Geometry: final body of the model. Coordinates: model frame, mm. A direction names the side the tool comes from. Coordinates: 2 decimals unless noted, no trailing zeros. Loops run counter-clockwise (first coordinate to the right, second up) from the corner with the lowest first, then second, coordinate; pieces in that order, holes last. Notation, with made-up numbers: (64, 73.5) -> (116, 73.5) arc R18 cw to (116, 77.5) -> close; hole circle Ø11 at (13, 89). An arc over 180 degrees is marked (long way). One line per item, written item: value. Start each with the question number.
from build123d import *

# Parameters (mm, degrees)
BOSS_EXTRUDE1_DEPTH                                  = 38.1
CBORE_FOR_3_8_BINDING_HEAD_MACHINE_SCREW_D           = 10.0838
CBORE_FOR_3_8_BINDING_HEAD_MACHINE_SCREW_CBORE_D     = 20.6375
CBORE_FOR_3_8_BINDING_HEAD_MACHINE_SCREW_CBORE_DEPTH = 3.175
FILLET1_R                                            = 2.54
FILLET2_R                                            = 6.35


with BuildPart() as part:
    # Sketch1 → Boss-Extrude1 (new body)
    with BuildSketch(Plane.XY):
        Polygon((0, 0), (44.45, 0), (44.45, -9.525), (-38.1608076, -9.525), (-38.1608076, 0), (-12.7608076, 0), (-6.35, 44.45), (0, 44.45), align=None)
    extrude(amount=BOSS_EXTRUDE1_DEPTH)

    # CBORE for 3/8 Binding Head Machine Screw1 (through all)
    with Locations(Plane(origin=(0, 0, 0), x_dir=(1, 0, 0), z_dir=(0, 1, 0))):
        with Locations((-25.4608076, -19.05)):
            CounterBoreHole(CBORE_FOR_3_8_BINDING_HEAD_MACHINE_SCREW_D / 2, CBORE_FOR_3_8_BINDING_HEAD_MACHINE_SCREW_CBORE_D / 2, CBORE_FOR_3_8_BINDING_HEAD_MACHINE_SCREW_CBORE_DEPTH)

    # Fillet1
    fillet1_edges = [part.edges().sort_by_distance(p)[0] for p in [
        (-12.7608076, 0, 19.05),
    ]]
    fillet(fillet1_edges, radius=FILLET1_R)

    # Fillet2
    fillet2_edges = [part.edges().sort_by_distance(p)[0] for p in [
        (0, 0, 19.05),
    ]]
    fillet(fillet2_edges, radius=FILLET2_R)


solid = part.part
1. Draft query along Z for faces 5 (the face through (0, 4, 38.1)), 6 (the face through (1.81, 1.91, 19.32)), 7 (the face through (-27.79, -6.39, 23.52)). Return one class per face: released by +Z, released by -Z, zero draft, split by the parting line, or undercut.
2. Section A-A on z = 19.05. Return the cut outline in (x, y) (3 decimals).
3. Line query: L1, parallel to X at y = -4.5, z = 19.05; L2, parallel to X at y = -3, z = 19; L3, parallel to Y at x = 10, z = 14.5 (3 decimals). Output: solid intervals per line, ascending. Write a range as [from, to].
4. Section B-B on z = 35.5. Return the cut outline in (x, y) (3 decimals).
5. Set-up query: faces 1 (the face through (-38.161, -5, 19)), 2 (the face through (-27.698, -1.565, 29.123)), 3 (the face through (0, 26, 19)), 4 (the face through (-37, 0, 19)). Return all of +Z, -Z, +X, -X, +Y, -Y with unobstructed straight access to the full face (end or side cutting, diameter ignored); none if empty.
6. Pin query (flat end, axial travel): pin 1 Ø18.5 at (x, z) = (-32, 15) entering from +Y; pin 2 Ø9 at (x, z) = (-25.46, 19.05) entering from -Y; pin 3 Ø1.5 at (y, z) = (3, 7) entering from -X; pin 4 Ø4 at (y, z) = (18.5, 21) entering from +X. Return the tip coordinate at first contact, or that it passes through.
7. Section D-D on y = 18.5. Return the cut outline in (x, z), plus the area to 3 significant figures.
8. Section C-C on x = 22. Return the cut outline in (y, z) (3 decimals).
Checks:
1. face 5: released by +Z
1. face 6: zero draft
1. face 7: undercut
2. outline: (-38.161, -9.525) -> (-30.503, -9.525) -> (-30.503, -3.175) -> (-35.78, -3.175) -> (-35.78, 0) -> (-38.161, 0) -> close; (-20.419, -9.525) -> (44.45, -9.525) -> (44.45, 0) -> (6.35, 0) arc R6.35 cw to (0, 6.35) -> (0, 44.45) -> (-6.35, 44.45) -> (-12.447, 2.177) arc R2.54 cw to (-14.961, 0) -> (-15.142, 0) -> (-15.142, -3.175) -> (-20.419, -3.175) -> close
3. L1: [-38.16, -30.5], [-20.42, 44.45]
3. L2: [-38.16, -35.78], [-15.14, 44.45]
3. L3: [-9.525, 0]
4. outline: (-38.161, -9.525) -> (44.45, -9.525) -> (44.45, 0) -> (6.35, 0) arc R6.35 cw to (0, 6.35) -> (0, 44.45) -> (-6.35, 44.45) -> (-12.447, 2.177) arc R2.54 cw to (-14.961, 0) -> (-38.161, 0) -> close
5. face 1: +Z, -Z, -X, +Y, -Y
5. face 2: +Y
5. face 3: +Z, -Z, +X, +Y
5. face 4: +Z, -Z, -X, +Y
6. pin 1: y = 0
6. pin 2: through
6. pin 3: x = -12.44
6. pin 4: x = 0
7. outline: (-10.09, 0) -> (0, 0) -> (0, 38.1) -> (-10.09, 38.1) -> close
7. area: 385 mm²
8. outline: (-9.525, 0) -> (0, 0) -> (0, 38.1) -> (-9.525, 38.1) -> close
